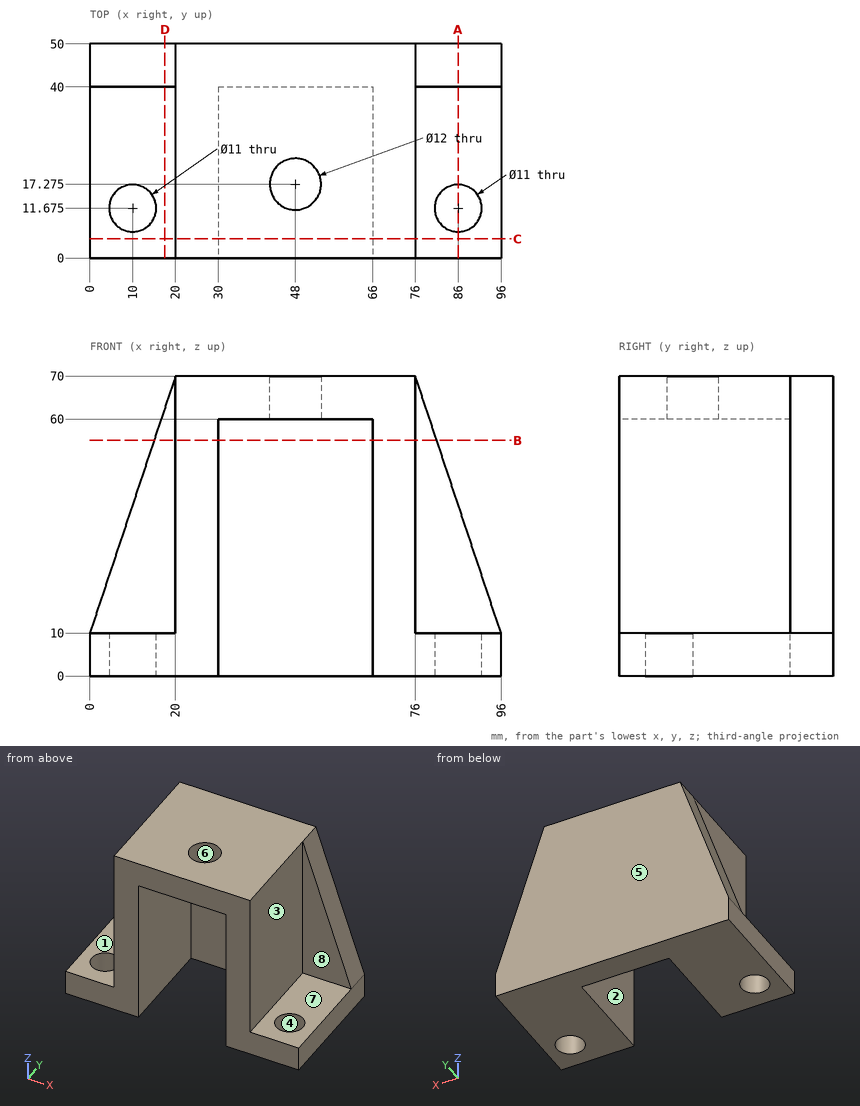
Job drawing, mm, ordinate dimensions from the low corner. One solid piece. A direction names the side the tool comes from. Give positions to 0.01 mm unless a question says otherwise; leave off trailing zeros. Write each loop counter-clockwise with the first axis right and the second up, starting at its lowest first coordinate (ties: lowest second). Pieces come first, ordered by that corner, then holes. Notation, with made-up numbers: (70.5, 65) -> (104.5, 65) arc R15 cw to (104.5, 73) -> close; hole circle Ø7 at (13, -27.75). An arc over 180 degrees is marked (long way). Return JSON: item names as keys, results as strings.
Item 1: Drill centre lines: probe 1 along X at (y, z) = (21, 44); probe 2 along Y at (x, z) = (86, 3.25) (3 decimals); probe 3 along Y at (x, z) = (48, 62) (3 decimals). Where is each one in solid material? Low to high.
Answer below:
{"probe 1": "x = 20 to 30, 66 to 76", "probe 2": "y = 0 to 6.175, 17.175 to 50", "probe 3": "y = 0 to 11.275, 23.275 to 50"}
Item 2: Tool access for the marked faces 1, 2, 3, 4 and 5: list every direction of +Z, -Z, +X, -X, +Y, -Y with a clear straight run to the whole face (end or side of a thin tool).
Answer below:
{"face 1": "+Z, -X, -Y", "face 2": "-Z, -Y", "face 3": "+Z, +X, -Y", "face 4": "+Z, -Z", "face 5": "+Z, -Z, +X, -X, +Y"}
Item 3: Band-saw the part on D-D (x = 17.5). List the corners of the cut face in (y, z).
Answer below:
{"outline": "(0, 0) -> (50, 0) -> (50, 62.5) -> (40, 62.5) -> (40, 10) -> (0, 10) -> close"}
Item 4: Drop flat-ended pins along their axis: pin 1 (3 mm diameter, centred on x = 54, z = 31.5, fed in from -Y); pin 2 (12 mm diameter, centred on y = 26.5, z = 16.5, fed in from +X); pin 3 (17.5 mm diameter, centred on x = 86, y = 11.675, fed in from +Z). Give the stop position or say it passes through.
Answer below:
{"pin 1": "stops at y = 40", "pin 2": "stops at x = 76", "pin 3": "stops at z = 10"}
Item 5: Band-saw the part on C-C (y = 4.5). List the corners of the cut face in (x, z), then the cut area to 3 significant figures.
Answer below:
{"outline": "(0, 0) -> (30, 0) -> (30, 60) -> (66, 60) -> (66, 0) -> (96, 0) -> (96, 10) -> (76, 10) -> (76, 70) -> (20, 70) -> (20, 10) -> (0, 10) -> close", "area": "2,160 mm2"}
Item 6: Band-saw the part on B-B (z = 55). List the corners of the cut face in (x, y).
Answer below:
{"outline": "(15, 40) -> (20, 40) -> (20, 0) -> (30, 0) -> (30, 40) -> (66, 40) -> (66, 0) -> (76, 0) -> (76, 40) -> (81, 40) -> (81, 50) -> (15, 50) -> close"}
Item 7: Band-saw the part on A-A (x = 86). List the corners of the cut face in (y, z) (3 decimals).
Answer below:
{"outline": "(0, 0) -> (6.175, 0) -> (6.175, 10) -> (0, 10) -> close; (17.175, 0) -> (50, 0) -> (50, 40) -> (40, 40) -> (40, 10) -> (17.175, 10) -> close"}
Item 8: Two-plate mould, pull along Y, no slides. Class the marked faces 6, 7 and 8: +Y half, -Y half, draft (parallel to the pull), parting line (faces both ways), or undercut.
Answer below:
{"face 6": "undercut", "face 7": "draft", "face 8": "-Y half"}
